Could you check a few things on this model? Use its own coordinates, in mm. Face numbers are marked on the shaded views. A direction names the side the tool comes from. Give positions to 0.01 mm unless a question says otherwise; leave off trailing zeros. Write each question's results on one line, items separated by ' | '.
```python
from build123d import *

# Parameters (mm, degrees)
FORO_15_0_15_1_D               = 15
FORO_11_0_11_2_D               = 11
FORO_11_0_11_2_DEPTH           = 27.5
FORO_11_0_11_2_ON_FACE_2_D     = 11
FORO_11_0_11_2_ON_FACE_2_DEPTH = 27.5
FORO_7_0_7_1_D                 = 7
FORO_7_0_7_1_DEPTH             = 27.5
SMUSSO1_SIZE                   = 1


with BuildPart() as part:
    # Schizzo2 → Rivoluzione2 (revolve)
    with BuildSketch(Plane.XY, mode=Mode.PRIVATE) as rivoluzione2_sk:
        Polygon((0, 0), (0, -34), (27.5, -34), (27.5, -16), (40, -16), (40, -8), (44.5, -8), (44.5, 0), align=None)
    revolve(rivoluzione2_sk.sketch.rotate(Axis((0, 0, 0), (0, -1, 0)), 90), axis=Axis((0, 0, 0), (0, -1, 0)))

    # Foro Ø15.0 (15)-1 (through all)
    with Locations(Plane.ZX):
        with Locations((0, 0)):
            Hole(FORO_15_0_15_1_D / 2)

    # Foro Ø11.0 (11)-2
    with Locations(Plane(origin=(-27.499989687, -24.000114667, -0.023815764), x_dir=(0.00086602778, 0, -0.999999624998), z_dir=(-0.999999624998, 0, -0.00086602778))):
        with Locations((0, 0)):
            Hole(FORO_11_0_11_2_D / 2, depth=FORO_11_0_11_2_DEPTH)

    # Foro Ø11.0 (11)-2 on face 2
    with Locations(Plane(origin=(-27.461073612, -24.000080572, -0.023731809), x_dir=(0.00086602778, 0, -0.999999624998), z_dir=(-0.999999624998, 0, -0.00086602778))):
        with Locations((0, 0)):
            Hole(FORO_11_0_11_2_ON_FACE_2_D / 2, depth=FORO_11_0_11_2_ON_FACE_2_DEPTH)

    # Foro Ø7.0 (7)-1
    with Locations(Plane(origin=(13.75, -24, 23.815698604), x_dir=(0.866025403784, 0, -0.5), z_dir=(0.5, 0, 0.866025403784))):
        with Locations((0, 0)):
            foro_7_0_7_1 = Hole(FORO_7_0_7_1_D / 2, depth=FORO_7_0_7_1_DEPTH)

    # Specchia1: Foro Ø7.0 (7)-1 across plane
    add(foro_7_0_7_1.mirror(Plane.XY), mode=Mode.SUBTRACT)

    # Smusso1
    smusso1_edges = [part.edges().sort_by_distance(p)[0] for p in [
        (0, -8, -44.5),
        (0, -16, -40),
        (0, -34, -27.5),
    ]]
    chamfer(smusso1_edges, length=SMUSSO1_SIZE)


solid = part.part
```
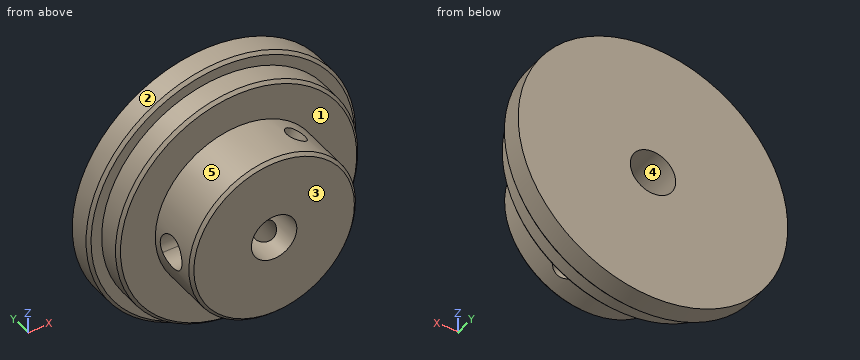
Q1. Thinking about a two-plate mould opening in X: for the marked faces 3, 4 and 5, which applies, +X half, -X half, draft (parallel to the pull), parting line (faces both ways), or undercut?
Here are the results:
face 3: draft | face 4: undercut | face 5: parting line
Q2. I need wall thicknesses on line 1 along Z through (x, y) = (0.5, -2); line 2 along X through (y, z) = (-17, 0); line 3 along Y through (x, z) = (20, -37.5). Which ranges of each line are inside material? Lowest first, please.
Here are the results:
line 1: z = -44.5 to -7.48, 7.48 to 44.5 | line 2: x = -27.5 to -7.5, 7.5 to 27.5 | line 3: y = -8 to 0
Q3. Suppose I cut it at A-A on z = 0. State how many separate pieces and enclosed holes the cut face has, and give its area (3 significant figures).
Here are the results:
separate pieces: 3 | enclosed holes: 0 | area: 1,610 mm²
Q4. For the marked faces 1 and 2, which set-ups out of +Z, -Z, +X, -X, +Y, -Y let a thin tool reach every point of the face, with its end or its side?
Here are the results:
face 1: -Y | face 2: +Y, -Y
Q5. I'm going to push flat-ended pins straight in: pin 1 Ø1.5 at (x, y) = (-5, -14) entering from +Z; pin 2 Ø10 at (y, z) = (-28, -18.5) entering from +X; pin 3 Ø10 at (x, y) = (32, -17) entering from -Z. Where does each tip first touch, or does it pass through?
Here are the results:
pin 1: stops at z = 39.77 | pin 2: stops at x = 23.96 | pin 3: stops at z = -29.13
